```python
from build123d import *

# Parameters (mm, degrees)
SKETCH2_R           = 1.30175
BOSS_EXTRUDE1_DEPTH = 9.525
CUT_EXTRUDE1_DEPTH  = 1.1176
CHAMFER1_SIZE       = 0.47244
FILLET1_R           = 0.254


with BuildPart() as part:
    # Sketch1 → Revolve1 (revolve)
    with BuildSketch(Plane.XY):
        with BuildLine():
            Line((1.5875, 1.4224), (0, 1.4224))
            Line((0, 1.4224), (0, 0))
            Line((0, 0), (2.235517502, 0))
            add(Edge.make_bspline(
                [(2.530228655, 0.381), (2.538792783, 0.348014811), (2.541780076, 0.313096126), (2.538943152, 0.279135577), (2.536106229, 0.245175028), (2.527366844, 0.211235941), (2.513448709, 0.180128827), (2.499530575, 0.149021713), (2.480049812, 0.119888598), (2.456619631, 0.09514201), (2.433189451, 0.070395421), (2.405163618, 0.049352817), (2.374862966, 0.033756745), (2.344562313, 0.018160672), (2.311151111, 0.007580973), (2.277396156, 0.002893755), (2.263536304, 0.000969174), (2.249510339, 0), (2.235517502, 0)],
                knots=[0, 0, 0, 0, 0.000102237, 0.000102237, 0.000102237, 0.000204473, 0.000204473, 0.000204473, 0.00030671, 0.00030671, 0.00030671, 0.000408946, 0.000408946, 0.000408946, 0.000511183, 0.000511183, 0.000511183, 0.000552664, 0.000552664, 0.000552664, 0.000552664], degree=3))
            ThreePointArc((2.530228655, 0.381), (2.18675257, 1.017470992), (1.5875, 1.4224))
        make_face()
    revolve(axis=Axis((0, 1.4224, 0), (0, -1, 0)))

    # Sketch2 → Boss-Extrude1 (add)
    with BuildSketch(Plane.XZ):
        Circle(SKETCH2_R)
    extrude(amount=BOSS_EXTRUDE1_DEPTH)

    # Sketch3 → Cut-Extrude1 (cut)
    with BuildSketch(Plane(origin=(0, 1.4224, 0), x_dir=(-1, 0, 0), z_dir=(0, 1, 0))):
        Polygon((0.536575, -0.929375162), (1.07315, 0), (0.536575, 0.929375162), (-0.536575, 0.929375162), (-1.07315, 0), (-0.536575, -0.929375162), align=None)
    extrude(amount=-CUT_EXTRUDE1_DEPTH, mode=Mode.SUBTRACT)

    # Chamfer1
    chamfer1_edges = [part.edges().sort_by_distance(p)[0] for p in [
        (-1.30175, -9.525, 0),
    ]]
    chamfer(chamfer1_edges, length=CHAMFER1_SIZE)

    # Fillet1
    fillet1_edges = [part.edges().sort_by_distance(p)[0] for p in [
        (-1.30175, 0, 0),
    ]]
    fillet(fillet1_edges, radius=FILLET1_R)


solid = part.part
```
Geometry: final body of the model. Coordinates: model frame, mm. A direction names the side the tool comes from. Coordinates: 2 decimals unless noted, no trailing zeros. Order: outer loops, then holes, each group sorted by start corner. A loop starts at its lowest first (then second) coordinate and runs counter-clockwise, first axis right, second up. Notation, with made-up numbers: M 25,-30 L 31,-30 A20 cw 31,-12 Z; hole C 83.5,10 d10. An arc over 180 degrees is marked long. Answer as CSV lines item,"result".
Q1. Draft query along X for faces 4 (the flat face through (0.809, 0.871, -0.458)), 5 (the cylindrical face through (1.24, -4.59, 0.39)), 6 (the flat face through (1, 1.422, -1)). Return one class per face: pulls with the +X half, pulls with the -X half, needs draft (parallel to the pull), parting line crosses it, or undercut.
Answers:
face 4,"undercut"
face 5,"parting line crosses it"
face 6,"needs draft"
Q2. Line query: probe 1 along Y at (x, z) = (-0.75, -1.35); probe 2 along Z at (x, y) = (0, -1.5); probe 3 along X at (y, z) = (-9, 0.75). Output: solid intervals per line, ascending. Write a range as [from, to].
Answers:
probe 1,"y = [0, 1.42]"
probe 2,"z = [-1.3, 1.3]"
probe 3,"x = [-1.06, 1.06]"
Q3. Section A-A on y = -8. Return the cut outline in (x, z), and give its area (3 significant figures).
Answers:
outline,"C 0,0 d2.6"
area,"5.32 mm^2"
Q4. First-contact query: P1, Ø1, axis at y = -8, z = 1, coming from the +X side; P2, Ø1.2, axis at x = 0, y = 1, coming from the +Z side; P3, Ø2, axis at x = -0.5, z = 0, coming from the +Y side; P4, Ø2, axis at y = -5.5, z = -0.5, coming from the +X side. Flat tips, straight axial feed; report the tip coordinate or a pass-through.
Answers:
P1,"stops at x = 1.2"
P2,"stops at z = 2.53"
P3,"stops at y = 1.42"
P4,"stops at x = 1.3"
Q5. Set-up query: faces 1 (the flat face through (0, 0, 2)), 2 (the flat face through (0, 1, -0.929)), 3 (the flat face through (0, -9.525, 0)). Return all of +Z, -Z, +X, -X, +Y, -Y with unobstructed straight access to the full face (end or side cutting, diameter ignored); none if empty.
Answers:
face 1,"-Y"
face 2,"+Y"
face 3,"+Z, -Z, +X, -X, -Y"
